from build123d import *

# Parameters (mm, degrees)
F0_W           = 185
F0_H           = 175
F0_R           = 20
F1_DEPTH       = 8
F3_D           = 6.5
F4_D           = 20
F5_D           = 7
F7_DEPTH       = 25
F9_D           = 6.6
F9_CBORE_D     = 11.25
F9_CBORE_DEPTH = 6
F10_R          = 2.5


with BuildPart() as f1:
    # F0 (on Front) → F1 (new body)
    with BuildSketch(Plane.XZ):
        Rectangle(F0_W, F0_H)
        with Locations((-42.5, 0)):
            Circle(F0_R, mode=Mode.SUBTRACT)
    extrude(amount=F1_DEPTH)

    # F3 (through all)
    with Locations(Plane.XZ.offset(8)):
        with Locations((-82.5, 80), (-42.5, 80), (-42.5, 40), (-82.5, 40), (-82.5, -40), (-42.5, -40), (-42.5, -80), (-82.5, -80), (42.5, -80), (82.5, -80), (82.5, -40), (42.5, -40), (42.5, 40), (82.5, 40), (82.5, 80), (42.5, 80)):
            Hole(F3_D / 2)

    # F4 (through all)
    with Locations(Plane.XZ.offset(8)):
        with Locations((-27.5, -42), (-27.5, 42)):
            Hole(F4_D / 2)

    # F5 (through all)
    with Locations(Plane.XZ.offset(8)):
        with Locations((-10, 67.5), (-10, -67.5)):
            Hole(F5_D / 2)

    # F6 (on face) → F7 (cut)
    with BuildSketch(Plane.XZ.offset(8)):
        with BuildLine():
            Line((6, -79.81), (6, -74.81))
            ThreePointArc((6, -74.81), (2.5, -71.31), (-1, -74.81))
            Line((-1, -74.81), (-1, -79.81))
            ThreePointArc((-1, -79.81), (2.5, -83.31), (6, -79.81))
        make_face()
        with BuildLine():
            Line((36, -79.81), (36, -74.81))
            ThreePointArc((36, -74.81), (32.5, -71.31), (29, -74.81))
            Line((29, -74.81), (29, -79.81))
            ThreePointArc((29, -79.81), (32.5, -83.31), (36, -79.81))
        make_face()
    extrude(amount=-F7_DEPTH, mode=Mode.SUBTRACT)

    # F9 (through all)
    with Locations(Plane(origin=(0, 0, 0), x_dir=(-1, 0, 0), z_dir=(0, 1, 0))):
        with Locations((75, 67.5), (75, -67.5)):
            CounterBoreHole(F9_D / 2, F9_CBORE_D / 2, F9_CBORE_DEPTH)

    # F10
    f10_edges = [f1.edges().sort_by_distance(p)[0] for p in [
        (-92.5, -4, 87.5),
        (-92.5, -4, -87.5),
        (92.5, -4, -87.5),
        (92.5, -4, 87.5),
    ]]
    fillet(f10_edges, radius=F10_R)


solid = f1.part
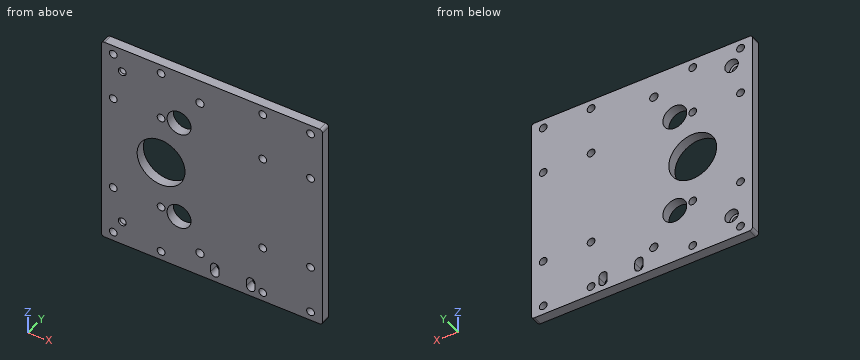
Geometry check sheet. Reference: the model listing, model coordinates, mm. Give positions to 0.01 mm unless a question says otherwise; leave off trailing zeros. Order: outer loops, then holes, each group sorted by start corner. A loop starts at its lowest first (then second) coordinate and runs counter-clockwise, first axis right, second up.
1) Cross-section at A-A (x = 42.5). Record the boundary of the cut face in (y, z).
Results are:
outline: (-8, -87.5) - (0, -87.5) - (0, -83.25) - (-8, -83.25) - close; (-8, -76.75) - (0, -76.75) - (0, -43.25) - (-8, -43.25) - close; (-8, -36.75) - (0, -36.75) - (0, 36.75) - (-8, 36.75) - close; (-8, 43.25) - (0, 43.25) - (0, 76.75) - (-8, 76.75) - close; (-8, 83.25) - (0, 83.25) - (0, 87.5) - (-8, 87.5) - close
2) Cross-section at C-C (z = -8). Record the boundary of the cut face in (x, y), then the cut area to 3 significant figures.
Results are:
outline: (-92.5, -8) - (-60.83, -8) - (-60.83, 0) - (-92.5, 0) - close; (-24.17, -8) - (92.5, -8) - (92.5, 0) - (-24.17, 0) - close
area: 1,190 mm2
3) Gauge pin test, flat end, axial feed: pin 1 (3.5 mm diameter, centred on x = -73, z = -67, fed in from +Y). Record the tip position at first contact, or that the pin passes through.
Results are:
pin 1: stops at y = -6
4) Cross-section at D-D (x = 2.5). Record the boundary of the cut face in (y, z), then the cut area to 3 significant figures.
Results are:
outline: (-8, -87.5) - (0, -87.5) - (0, -83.31) - (-8, -83.31) - close; (-8, -71.31) - (0, -71.31) - (0, 87.5) - (-8, 87.5) - close
area: 1,300 mm2
5) Material ranges on probe 1 along Z at (x, y) = (82.5, -2); probe 2 along Z at (x, y) = (-42.5, -4); probe 3 along Z at (x, y) = (-27.5, -4), recorded low to high.
Results are:
probe 1: z = -87.5 to -83.25, -76.75 to -43.25, -36.75 to 36.75, 43.25 to 76.75, 83.25 to 87.5
probe 2: z = -87.5 to -83.25, -76.75 to -43.25, -36.75 to -20, 20 to 36.75, 43.25 to 76.75, 83.25 to 87.5
probe 3: z = -87.5 to -52, -32 to -13.23, 13.23 to 32, 52 to 87.5
6) Cross-section at B-B (z = 80). Record the boundary of the cut face in (x, y).
Results are:
outline: (-92.5, -8) - (-85.75, -8) - (-85.75, 0) - (-92.5, 0) - close; (-79.25, -8) - (-45.75, -8) - (-45.75, 0) - (-79.25, 0) - close; (-39.25, -8) - (39.25, -8) - (39.25, 0) - (-39.25, 0) - close; (45.75, -8) - (79.25, -8) - (79.25, 0) - (45.75, 0) - close; (85.75, -8) - (92.5, -8) - (92.5, 0) - (85.75, 0) - close
